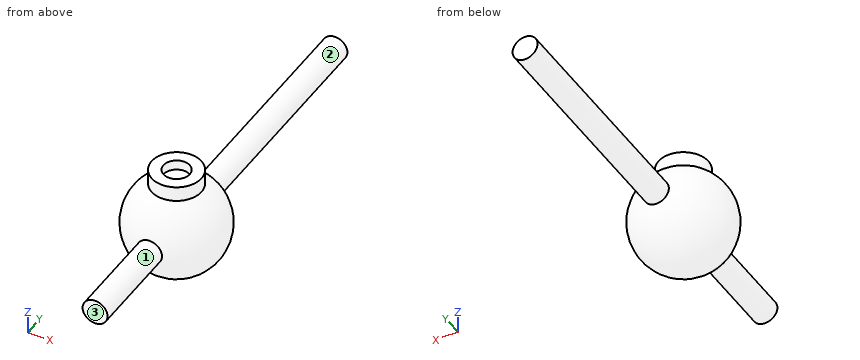
```python
from build123d import *

# Parameters (mm, degrees)
BOSS_EXTRUDE1_START = 7
SKETCH1_R           = 6
SKETCH1_R_2         = 3.175
BOSS_EXTRUDE1_DEPTH = 7


with BuildPart() as part:
    # Sketch1 → Boss-Extrude1 (new body)
    with BuildSketch(Plane.XY.offset(BOSS_EXTRUDE1_START)):
        Circle(SKETCH1_R)
        Circle(SKETCH1_R_2, mode=Mode.SUBTRACT)
    extrude(amount=BOSS_EXTRUDE1_DEPTH)

    # Sketch2 → Revolve1 (revolve)
    with BuildSketch(Plane.XY, mode=Mode.PRIVATE) as revolve1_sk:
        with BuildLine():
            Line((0, -35), (3, -35))
            Line((3, -35), (3, -11.618950039))
            ThreePointArc((3, -11.618950039), (12, 0), (3, 11.618950039))
            Line((3, 11.618950039), (3, 68))
            Line((3, 68), (0, 68))
            Line((0, 68), (0, -35))
        make_face()
    revolve(revolve1_sk.sketch.rotate(Axis((0, -35, 0), (0, 1, 0)), 90), axis=Axis((0, -35, 0), (0, 1, 0)))


solid = part.part
```
Work out the finished part from the listing and answer in its coordinate system (mm). Face numbers are marked on the shaded views. A direction names the side the tool comes from. Coordinates: 2 decimals unless noted, no trailing zeros. Loops run counter-clockwise (first coordinate to the right, second up) from the corner with the lowest first, then second, coordinate; pieces in that order, holes last.
1) For the marked faces 1, 2 and 3, determine the directions among +Z, -Z, +X, -X, +Y, -Y from which every point of the face is accessible in a straight line to the end or side of a thin tool.
Results:
face 1: -Y
face 2: +Y
face 3: +Z, -Z, +X, -X, -Y
2) Section C-C (x = 9.5) is taken. Give the vertices of the cut face in (y, z), plus the area to 3 significant figures.
Results:
outline: circle Ø14.66 at (0, 0)
area: 169 mm2
3) Consider probe 1 along X at (y, z) = (0, 12.2) (3 decimals); probe 2 along X at (y, z) = (-2, 12.5). Determine where each line is inside the solid, lowest interval first.
Results:
probe 1: x = -6 to -3.175, 3.175 to 6
probe 2: x = -5.66 to -2.47, 2.47 to 5.66
4) Section B-B (y = 0) is taken. Give the vertices of the cut face in (x, z) (3 decimals), plus the area to 3 significant figures.
Results:
outline: (-6, 10.392) arc R12 ccw (long way) to (6, 10.392) - (6, 14) - (3.175, 14) - (3.175, 11.572) arc R12 ccw to (-3.175, 11.572) - (-3.175, 14) - (-6, 14) - close
area: 469 mm2
5) Section D-D (y = 58) is taken. Give the vertices of the cut face in (x, z), plus the area to 3 significant figures.
Results:
outline: circle Ø6 at (0, 0)
area: 28.3 mm2
6) Flat-ended cylindrical pins translate along their axes: pin 1 (6 mm diameter, centred on y = -9, z = -6, fed in from -X); pin 2 (1 mm diameter, centred on x = 0, y = 22.5, fed in from +Z); pin 3 (8 mm diameter, centred on x = 8, y = 47, fed in from +Z); pin 4 (3 mm diameter, centred on x = 6, z = 7.5, fed in from -Y). Find the tip coordinate at first contact, or state that the pin passes through.
Results:
pin 1: stops at x = -9.1
pin 2: stops at z = 3
pin 3: passes through
pin 4: stops at y = -8.85
7) Section A-A (z = 0) is taken. Give the vertices of the cut face in (x, y).
Results:
outline: (-3, -35) - (3, -35) - (3, -11.62) arc R12 ccw to (3, 11.62) - (3, 68) - (-3, 68) - (-3, 11.62) arc R12 ccw to (-3, -11.62) - close
